Design review of the part shown in the three views and the two pictorial views. Dimensions are in mm from the part's minimum x, y and z. Round coordinates to 2 decimals unless told otherwise and drop trailing zeros. Order: outer loops, then holes, each group sorted by start corner. A loop starts at its lowest first (then second) coordinate and runs counter-clockwise, first axis right, second up. Notation, with made-up numbers: M -19.75,88.25 L 2.25,88.25 A19 ccw 2.25,100.25 Z; hole C 73,81.5 d7. An arc over 180 degrees is marked long. Write each question's results on one line, items separated by ' | '. Start each with the question number.
Item 1: Wall thickness on line 1 (Y direction, x = 39.92, z = 103); line 2 (Y direction, x = 39, z = 34): over which ranges is each line inside the solid? List them lowest first. Write a range as [from, to].
Item 2: Clearance check with flat-ended pins moving along their axes: pin 1 (8 mm diameter, centred on x = 23.5, z = 120, fed in from +Y); pin 2 (5 mm diameter, centred on x = 54, y = 56, fed in from +Z); pin 3 (8 mm diameter, centred on y = 28.5, z = 95, fed in from +X); pin 4 (4 mm diameter, centred on y = 61, z = 91.5, fed in from +X). State where each tip first meets the part, or that it passes through.
Item 3: The part is to be moulded in two halves that separate along X. For the marked faces 1, 2 and 3, say which applies: +X half, -X half, draft (parallel to the pull), parting line (faces both ways), or undercut.
Item 4: Take a section at A-A, the plane x = 39.92. Write out the cut boundary in (y, z).
Item 5: Take a section at C-C, the plane z = 121.5. Write out the cut boundary in (x, y), plus the area to 3 significant figures.
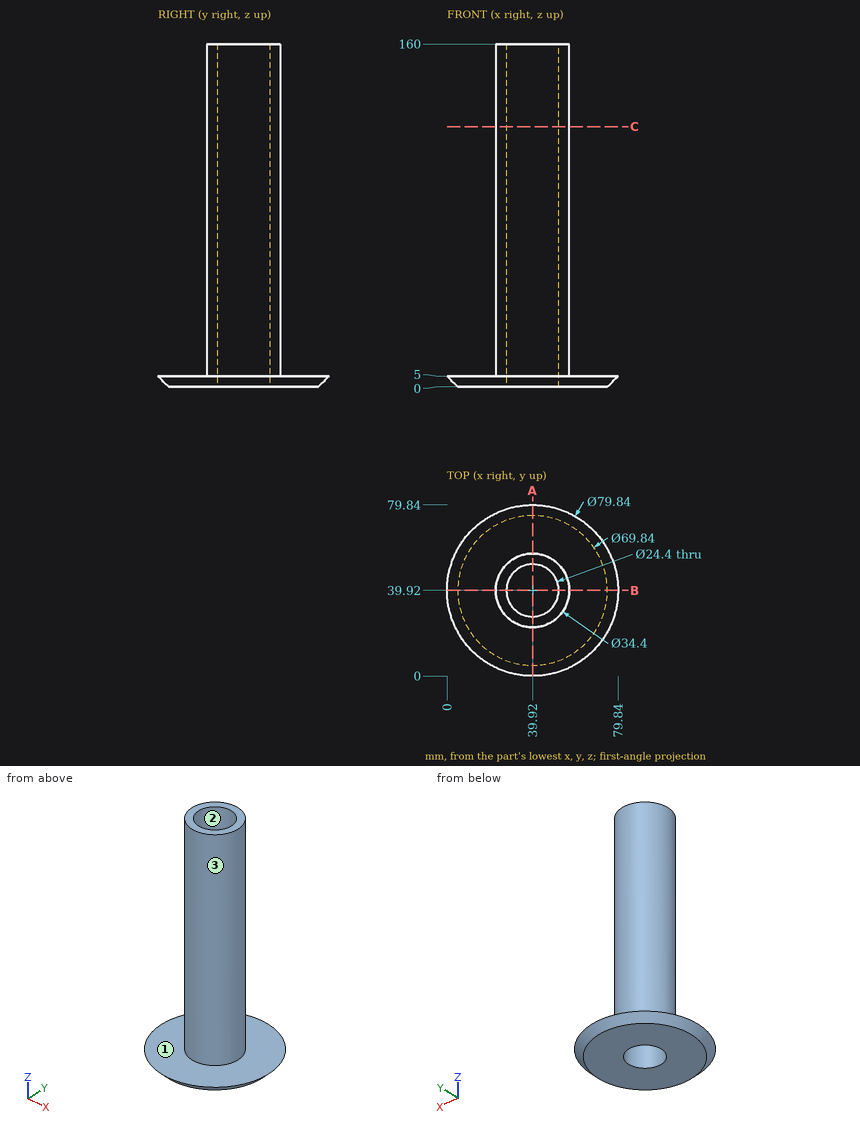
Results list:
1) line 1: [22.72, 27.72], [52.12, 57.12] | line 2: [22.74, 27.75], [52.09, 57.1]
2) pin 1: y = 51.82 | pin 2: z = 5 | pin 3: x = 55.44 | pin 4: through
3) face 1: draft | face 2: undercut | face 3: parting line
4) outline: M 0,5 L 5,0 L 27.72,0 L 27.72,160 L 22.72,160 L 22.72,5 Z; M 52.12,0 L 74.84,0 L 79.84,5 L 57.12,5 L 57.12,160 L 52.12,160 Z
5) outline: C 39.92,39.92 d34.4; hole C 39.92,39.92 d24.4 | area: 462 mm²
